```python
from build123d import *
from build123d.topology import SkipClean

# Parameters (mm, degrees)
BOSS_EXTRUDE1_DEPTH                              = 10
SKETCH3_R                                        = 9
BOSS_EXTRUDE2_DEPTH                              = 16
FILLET1_R                                        = 4
CHAMFER1_SIZE                                    = 2
BOSS_EXTRUDE3_START                              = 10
SKETCH5_R                                        = 13
BOSS_EXTRUDE3_DEPTH                              = 10
CUT_EXTRUDE1_DEPTH                               = 94.03897033
CUT_EXTRUDE1_DEPTH_BACK                          = 94.03897033
SKETCH4_R                                        = 9
CIRPATTERN1_COUNT                                = 3
CUT_EXTRUDE2_DEPTH                               = 94.03897033
CUT_EXTRUDE2_DEPTH_BACK                          = 94.03897033
SKETCH7_R                                        = 9
CBORE_FOR_M8_HEX_HEAD_MACHINE_SCREW1_D           = 9
CBORE_FOR_M8_HEX_HEAD_MACHINE_SCREW1_CBORE_D     = 15
CBORE_FOR_M8_HEX_HEAD_MACHINE_SCREW1_CBORE_DEPTH = 6
SKETCH11_W                                       = 3
SKETCH11_H                                       = 2
BOSS_EXTRUDE4_DEPTH                              = 5
CIRPATTERN2_COUNT                                = 3
SKETCH14_R                                       = 2.5
BOSS_EXTRUDE5_DEPTH                              = 10
BOSS_EXTRUDE6_START                              = -10
BOSS_EXTRUDE6_DEPTH                              = 10
SKETCH16_R                                       = 7.5
BOSS_EXTRUDE7_DEPTH                              = 21
CUT_EXTRUDE4_DEPTH                               = 112.813460728
CUT_EXTRUDE4_DEPTH_BACK                          = 112.813460728
SKETCH17_R                                       = 4
BOSS_EXTRUDE9_DEPTH                              = 3
CUT_EXTRUDE5_DEPTH                               = 3
CIRPATTERN3_COUNT                                = 3
FILLET6_R                                        = 10
FILLET7_R                                        = 10
FILLET8_R                                        = 10
FILLET9_R                                        = 10


with BuildPart() as part:
    # Sketch1 → Revolve1 (revolve)
    with BuildSketch(Plane.XY, mode=Mode.PRIVATE) as revolve1_sk:
        Polygon((0, 0), (50, 0), (50, -24), (45, -24), (45, -9), (0, -9), align=None)
    revolve(revolve1_sk.sketch.rotate(Axis((0, -30.388235294, 0), (0, 1, 0)), 90), axis=Axis((0, -30.388235294, 0), (0, 1, 0)))

    # Sketch2 → Boss-Extrude1 (add)
    with BuildSketch(Plane(origin=(0, 0, 0), x_dir=(1, 0, 0), z_dir=(0, 1, 0))):
        with BuildLine():
            Line((-48.412291828, 12.5), (-55, 12.5))
            ThreePointArc((-55, 12.5), (-67.5, 0), (-55, -12.5))
            Line((-55, -12.5), (-48.412291828, -12.5))
            Line((-48.412291828, -12.5), (-48.412291828, 12.5))
        make_face()
        with BuildLine():
            Line((48.412291828, -12.5), (48.412291828, 12.5))
            Line((48.412291828, 12.5), (55, 12.5))
            ThreePointArc((55, 12.5), (67.5, 0), (55, -12.5))
            Line((55, -12.5), (48.412291828, -12.5))
        make_face()
    extrude(amount=-BOSS_EXTRUDE1_DEPTH)

    # Sketch3 → Boss-Extrude2 (add)
    with BuildSketch(Plane(origin=(0, 0, 0), x_dir=(1, 0, 0), z_dir=(0, 1, 0))):
        with BuildLine():
            Line((32.04293994, -5.5), (11.258330249, 30.5))
            ThreePointArc((11.258330249, 30.5), (0, 37), (-11.258330249, 30.5))
            Line((-11.258330249, 30.5), (-32.04293994, -5.5))
            ThreePointArc((-32.04293994, -5.5), (-32.04293994, -18.5), (-20.784609691, -25))
            Line((-20.784609691, -25), (20.784609691, -25))
            ThreePointArc((20.784609691, -25), (32.04293994, -18.5), (32.04293994, -5.5))
        make_face()
        with Locations(Location((0, 24, 0), (0, 0, 270))):
            Circle(SKETCH3_R, mode=Mode.SUBTRACT)
        with Locations(Location((20.784609691, -12, 0), (0, 0, 270))):
            Circle(SKETCH3_R, mode=Mode.SUBTRACT)
        with Locations(Location((-20.784609691, -12, 0), (0, 0, 270))):
            Circle(SKETCH3_R, mode=Mode.SUBTRACT)
    extrude(amount=BOSS_EXTRUDE2_DEPTH)

    # Fillet1
    fillet1_edges = [part.edges().sort_by_distance(p)[0] for p in [
        (0, 0, -37),
        (-21.650635095, 0, -12.5),
        (-32.04293994, 0, 18.5),
        (0, 0, 25),
        (32.04293994, 0, 18.5),
        (21.650635095, 0, -12.5),
    ]]
    fillet(fillet1_edges, radius=FILLET1_R)

    # Chamfer1
    chamfer1_edges = [part.edges().sort_by_distance(p)[0] for p in [
        (20.784609691, 16, 3),
        (0, 16, -33),
        (-20.784609691, 16, 3),
    ]]
    chamfer(chamfer1_edges, length=CHAMFER1_SIZE)

    # Sketch5 → Boss-Extrude3 (add)
    with BuildSketch(Plane.XZ.offset(9).offset(BOSS_EXTRUDE3_START)):
        with Locations(Location((-20.784609691, 12, 0), (0, 0, 270))):
            Circle(SKETCH5_R)
    boss_extrude3 = extrude(amount=-BOSS_EXTRUDE3_DEPTH)

    # Sketch4 → Cut-Extrude1 (cut, two sides: drawn at the far end of the back side and taken through both)
    with SkipClean():  # the faces are left unmerged after this step: merging them gives an invalid solid
        with BuildSketch(Plane(origin=(0, 16, 0), x_dir=(1, 0, 0), z_dir=(0, 1, 0)).offset(-CUT_EXTRUDE1_DEPTH_BACK)):
            with Locations(Location((0, 24, 0), (0, 0, 90))):
                Circle(SKETCH4_R)
            with Locations(Location((20.784609691, -12, 0), (0, 0, 90))):
                Circle(SKETCH4_R)
            with Locations(Location((-20.784609691, -12, 0), (0, 0, 90))):
                Circle(SKETCH4_R)
        extrude(amount=CUT_EXTRUDE1_DEPTH + CUT_EXTRUDE1_DEPTH_BACK, mode=Mode.SUBTRACT)

    # CirPattern1: Boss-Extrude3 ×3 about axis
    with SkipClean():  # the faces are left unmerged after this step: merging them gives an invalid solid
        cirpattern1_axis = Axis((0, 0, 0), (0, 1, 0))
        for i in range(1, CIRPATTERN1_COUNT):
            add(boss_extrude3.rotate(cirpattern1_axis, i * 360 / CIRPATTERN1_COUNT))

    # Sketch7 → Cut-Extrude2 (cut, two sides: drawn at the far end of the back side and taken through both)
    with SkipClean():  # the faces are left unmerged after this step: merging them gives an invalid solid
        with BuildSketch(Plane(origin=(0, 16, 0), x_dir=(1, 0, 0), z_dir=(0, 1, 0)).offset(-CUT_EXTRUDE2_DEPTH_BACK)):
            with Locations(Location((0, 24, 0), (0, 0, 90))):
                Circle(SKETCH7_R)
            with Locations(Location((20.784609691, -12, 0), (0, 0, 90))):
                Circle(SKETCH7_R)
        extrude(amount=CUT_EXTRUDE2_DEPTH + CUT_EXTRUDE2_DEPTH_BACK, mode=Mode.SUBTRACT)

    # CBORE for M8 Hex Head Machine Screw1 (through all)
    with Locations(Plane(origin=(0, 0, 0), x_dir=(1, 0, 0), z_dir=(0, 1, 0))):
        with Locations((-55, 0), (55, 0)):
            CounterBoreHole(CBORE_FOR_M8_HEX_HEAD_MACHINE_SCREW1_D / 2, CBORE_FOR_M8_HEX_HEAD_MACHINE_SCREW1_CBORE_D / 2, CBORE_FOR_M8_HEX_HEAD_MACHINE_SCREW1_CBORE_DEPTH)

    # Sketch11 → Cut-Revolve1 (revolve, cut)
    with SkipClean():  # the faces are left unmerged after this step: merging them gives an invalid solid
        with BuildSketch(Plane.XY, mode=Mode.PRIVATE) as cut_revolve1_sk:
            with Locations((-48.5, -17)):
                Rectangle(SKETCH11_W, SKETCH11_H)
            with Locations((-48.5, -21)):
                Rectangle(SKETCH11_W, SKETCH11_H)
        revolve(cut_revolve1_sk.sketch.rotate(Axis((0, 0, 0), (0, -1, 0)), 270), axis=Axis((0, 0, 0), (0, -1, 0)), mode=Mode.SUBTRACT)

    # Sketch12 → Boss-Extrude4 (add, symmetric)
    with SkipClean():  # the faces are left unmerged after this step: merging them gives an invalid solid
        with BuildSketch(Plane(origin=(0, 0, 0), x_dir=(0, 0, -1), z_dir=(1, 0, 0))):
            Polygon((-25, 10), (-31.339745962, 10), (-40, 5), (-40, 0), (-25, 0), align=None)
        boss_extrude4 = extrude(amount=BOSS_EXTRUDE4_DEPTH, both=True)

    # CirPattern2: Boss-Extrude4 ×3 about axis
    with SkipClean():  # the faces are left unmerged after this step: merging them gives an invalid solid
        cirpattern2_axis = Axis((0, 0, 0), (0, 1, 0))
        for i in range(1, CIRPATTERN2_COUNT):
            add(boss_extrude4.rotate(cirpattern2_axis, i * 360 / CIRPATTERN2_COUNT))

    # Sketch14 → Boss-Extrude5 (add)
    with SkipClean():  # the faces are left unmerged after this step: merging them gives an invalid solid
        with BuildSketch(Plane(origin=(10, 0, 0), x_dir=(0, 0, -1), z_dir=(1, 0, 0))):
            with BuildLine():
                Line((-60, 0), (-45, 0))
                Line((-45, 0), (-45, -10))
                Line((-45, -10), (-60, -10))
                ThreePointArc((-60, -10), (-65, -5), (-60, 0))
            make_face()
            with Locations((-60, -5)):
                Circle(SKETCH14_R, mode=Mode.SUBTRACT)
        boss_extrude5 = extrude(amount=BOSS_EXTRUDE5_DEPTH)

    # Mirror1: Boss-Extrude5 across plane
    with SkipClean():  # the faces are left unmerged after this step: merging them gives an invalid solid
        add(boss_extrude5.mirror(Plane(origin=(0, 0, 0), x_dir=(0, 0, 1), z_dir=(1, 0, 0))))

    # Sketch15 → Boss-Extrude6 (add)
    with SkipClean():  # the faces are left unmerged after this step: merging them gives an invalid solid
        with BuildSketch(Plane(origin=(0, 0, 0), x_dir=(1, 0, 0), z_dir=(0, 1, 0)).offset(BOSS_EXTRUDE6_START)):
            with BuildLine():
                Line((-25, 43.301270189), (-25, 60))
                ThreePointArc((-25, 60), (0, 65), (25, 60))
                Line((25, 60), (25, 43.301270189))
                ThreePointArc((25, 43.301270189), (0, 50), (-25, 43.301270189))
            make_face()
            with BuildLine():
                ThreePointArc((18.541019662, 57.063390978), (0, 60), (-18.541019662, 57.063390978))
                ThreePointArc((-18.541019662, 57.063390978), (-20.146118467, 53.913207201), (-16.995934691, 52.308108396))
                ThreePointArc((-16.995934691, 52.308108396), (0, 55), (16.995934691, 52.308108396))
                ThreePointArc((16.995934691, 52.308108396), (20.146118467, 53.913207201), (18.541019662, 57.063390978))
            make_face(mode=Mode.SUBTRACT)
        extrude(amount=BOSS_EXTRUDE6_DEPTH)

    # Sketch16 → Boss-Extrude7 (add)
    with SkipClean():  # the faces are left unmerged after this step: merging them gives an invalid solid
        with BuildSketch(Plane(origin=(0, 16, 0), x_dir=(1, 0, 0), z_dir=(0, 1, 0))):
            with Locations(Location((0, 0, 0), (0, 0, 90))):
                Circle(SKETCH16_R)
        extrude(amount=BOSS_EXTRUDE7_DEPTH)

    # Sketch17 → Cut-Extrude4 (cut, two sides: drawn at the far end of the back side and taken through both)
    with SkipClean():  # the faces are left unmerged after this step: merging them gives an invalid solid
        with BuildSketch(Plane(origin=(0, 37, 0), x_dir=(1, 0, 0), z_dir=(0, 1, 0)).offset(-CUT_EXTRUDE4_DEPTH_BACK)):
            with Locations(Location((0, 0, 0), (0, 0, 270))):
                Circle(SKETCH17_R)
        extrude(amount=CUT_EXTRUDE4_DEPTH + CUT_EXTRUDE4_DEPTH_BACK, mode=Mode.SUBTRACT)

    # Sketch19 → Boss-Extrude9 (add, symmetric)
    with SkipClean():  # the faces are left unmerged after this step: merging them gives an invalid solid
        with BuildSketch(Plane(origin=(0, 0, 0), x_dir=(0, 0, -1), z_dir=(1, 0, 0))):
            with BuildLine():
                Line((-5.5, 37), (-15, 37))
                ThreePointArc((-15, 37), (-18.535533906, 35.535533906), (-20, 32))
                Line((-20, 32), (-20, 15.631109771))
                Line((-20, 15.631109771), (-17, 15.631109771))
                Line((-17, 15.631109771), (-17, 32))
                ThreePointArc((-17, 32), (-16.414213562, 33.414213562), (-15, 34))
                Line((-15, 34), (-5.5, 34))
                Line((-5.5, 34), (-5.5, 37))
            make_face()
        boss_extrude9 = extrude(amount=BOSS_EXTRUDE9_DEPTH, both=True)

    # Sketch21 → Cut-Extrude5 (cut, symmetric)
    with SkipClean():  # the faces are left unmerged after this step: merging them gives an invalid solid
        with BuildSketch(Plane(origin=(0, 0, 0), x_dir=(0, 0, -1), z_dir=(1, 0, 0))):
            with BuildLine():
                Line((-17, 16), (-17, 32))
                ThreePointArc((-17, 32), (-16.414213562, 33.414213562), (-15, 34))
                Line((-15, 34), (-6.873863542, 34))
                Line((-6.873863542, 34), (-6.873863542, 16))
                Line((-6.873863542, 16), (-17, 16))
            make_face()
        cut_extrude5 = extrude(amount=CUT_EXTRUDE5_DEPTH, both=True, mode=Mode.SUBTRACT)

    # CirPattern3: Boss-Extrude9, Cut-Extrude5 ×3 about axis
    with SkipClean():  # the faces are left unmerged after this step: merging them gives an invalid solid
        cirpattern3_axis = Axis((0, 0, 0), (0, 1, 0))
        add([boss_extrude9.rotate(cirpattern3_axis, i * 360 / CIRPATTERN3_COUNT) for i in range(1, CIRPATTERN3_COUNT)])
        add([cut_extrude5.rotate(cirpattern3_axis, i * 360 / CIRPATTERN3_COUNT) for i in range(1, CIRPATTERN3_COUNT)], mode=Mode.SUBTRACT)

    # Fillet6
    fillet6_edges = [part.edges().sort_by_distance(p)[0] for p in [
        (25, -5, -43.301270189),
    ]]
    fillet(fillet6_edges, radius=FILLET6_R)

    # Fillet7
    fillet7_edges = [part.edges().sort_by_distance(p)[0] for p in [
        (25, -5, -60),
    ]]
    fillet(fillet7_edges, radius=FILLET7_R)

    # Fillet8
    fillet8_edges = [part.edges().sort_by_distance(p)[0] for p in [
        (-25, -5, -60),
    ]]
    fillet(fillet8_edges, radius=FILLET8_R)

    # Fillet9
    fillet9_edges = [part.edges().sort_by_distance(p)[0] for p in [
        (-25, -5, -43.301270189),
    ]]
    fillet(fillet9_edges, radius=FILLET9_R)


solid = part.part
```
Geometry: final body of the model. Coordinates: model frame, mm. A direction names the side the tool comes from. Give positions to 0.01 mm unless a question says otherwise; leave off trailing zeros. Write each loop counter-clockwise with the first axis right and the second up, starting at its lowest first coordinate (ties: lowest second). Pieces come first, ordered by that corner, then holes.
1. Draft query along Y for faces 5 (the cylindrical face through (-14.93, -5.96, 57.69)), 6 (the flat face through (-20, -5, 53)), 7 (the flat face through (4.2, 37, -1.2)), 8 (the flat face through (33, -20, -34)). Return one class per face: released by +Y, released by -Y, zero draft, split by the parting line, or undercut.
2. Line query: probe 1 along Z at (x, y) = (23, -11); probe 2 along Z at (x, y) = (-31, -10.5); probe 3 along X at (y, z) = (1, 12). Output: solid intervals per line, ascending.
3. Section query A-A, the plane y = 23. Return loops of the section in (x, z) (1 decimal), then the cut area to 3 significant figures.
4. Reachability of faces 1 (the flat face through (17.3, 24.112, -10.036)), 2 (the cylindrical face through (-15.02, -23.01, -47.69)), 3 (the flat face through (33, -16, -34)), 4 (the flat face through (-52, -5, 12.5)) from +Z, -Z, +X, -X, +Y, -Y: full face, straight path, thin tool, end or side. Return the list, or none.
5. Pin query (flat end, axial travel): P1, Ø8, axis at x = 1.5, z = -24.5, coming from the -Y side; P2, Ø3, axis at y = -7.5, z = 59, coming from the +X side; P3, Ø7.5, axis at x = -7.5, z = -6.5, coming from the -Y side; P4, Ø3.5, axis at x = 52, y = -4, coming from the -Z side. Return the tip coordinate at first contact, or that it passes through.
6. Section query C-C, the plane y = -12. Return loops of the section in (x, z).
7. Section query B-B, the plane x = 0. Count the separate pieces of the cut face and the enclosed holes in it, then the cut area to 3 significant figures.
8. Section query D-D, the plane z = 37. Return loops of the section in (x, y), then the cut area to 3 significant figures.
Computed:
1. face 5: undercut
1. face 6: zero draft
1. face 7: released by +Y
1. face 8: undercut
2. probe 1: z = -44.4 to -38.68, -0.81 to 3.28, 20.72 to 24.81, 38.68 to 44.4
2. probe 2: z = -39.23 to -32.62, 3.96 to 20.04, 32.62 to 39.23
2. probe 3: x = -35.14 to -29.78, -11.78 to 11.78, 29.78 to 35.14
3. outline: (-18.8, -7.4) - (-15.8, -12.6) - (-13.2, -11.1) - (-16.2, -5.9) - close; (-7.5, -0.8) - (-4.5, -6) arc R7.5 ccw to (4.5, -6) - (7.5, -0.8) arc R7.5 ccw to (3, 6.9) - (-3, 6.9) arc R7.5 ccw to start; (-3, 17) - (3, 17) - (3, 20) - (-3, 20) - close; (13.2, -11.1) - (15.8, -12.6) - (18.8, -7.4) - (16.2, -5.9) - close; hole circle Ø8 at (0, 0)
3. area: 173 mm2
4. face 1: -Z, +X, +Y
4. face 2: -Y
4. face 3: none
4. face 4: +Z, -X, +Y, -Y
5. P1: passes through
5. P2: stops at x = 20
5. P3: stops at y = -9
5. P4: stops at z = -12.5
6. outline: circle Ø100 at (0, 0); circle Ø26 at (-20.78, 12); circle Ø26 at (0, -24); circle Ø26 at (20.78, 12); hole circle Ø90 at (0, 0); hole circle Ø18 at (-20.78, 12); hole circle Ø18 at (0, -24); hole circle Ø18 at (20.78, 12)
7. separate pieces: 4
7. enclosed holes: 1
7. area: 1,900 mm2
8. outline: (-33.63, -24) - (-25.61, -24) - (-25.61, -9) - (25.61, -9) - (25.61, -24) - (33.63, -24) - (33.63, -22) - (28.98, -22) - (28.98, -20) - (33.63, -20) - (33.63, -18) - (28.98, -18) - (28.98, -16) - (33.63, -16) - (33.63, 0) - (5, 0) - (5, 6.73) - (-5, 6.73) - (-5, 0) - (-33.63, 0) - (-33.63, -16) - (-28.98, -16) - (-28.98, -18) - (-33.63, -18) - (-33.63, -20) - (-28.98, -20) - (-28.98, -22) - (-33.63, -22) - close
8. area: 876 mm2
